Autodesk Inventor part; units mm, degrees
ref_plane "YZ Plane" through (0, 0, 0) normal (1, 0, 0) x (0, 1, 0)
ref_plane "XZ Plane" through (0, 0, 0) normal (0, 1, 0) x (-1, 0, 0)
ref_plane "XY Plane" through (0, 0, 0) normal (0, 0, 1) x (1, 0, 0)
sketch "Sketch1" plane through (0, 0, 0) normal (0, 0, 1) x (1, 0, 0)
  arc A0 (0, 12.7) -> (0, -12.7) centre (0, 0) ccw
  line L0 (0, 12.7) -> (17.145, 12.7)
  line L1 (17.145, 12.7) -> (17.145, -12.7)
  line L2 (17.145, -12.7) -> (0, -12.7)
  line L3 (0, -12.7) -> (0, 12.7)
  dimension "d0" = 25.4
  dimension "d7" = 17.145
extrude "Extrusion1" add sketch "Sketch1" along normal blind 4
sketch "Sketch2" plane through (0, 0, 4) normal (0, 0, 1) x (1, 0, 0)
  circle A0 centre (0, 0) radius 2.75
  dimension "d4" = 5.5
extrude "Extrusion2" cut sketch "Sketch2" against normal through all
sketch "Sketch3" plane through (17.145, -12.7, 0) normal (1, 0, 0) x (0, 0, -1)
  line L0 (-9.3431, 3.937) -> (-2.54, 3.937)
  line L1 (4.3638, 3.937) -> (4.3638, 21.463)
  line L2 (4.3638, 21.463) -> (0, 21.463)
  line L3 (-9.3431, 21.463) -> (-9.3431, 3.937)
  arc A0 (-2.54, 3.937) -> (0, 3.937) centre (-1.27, 3.937) ccw
  arc A1 (0, 21.463) -> (-2.54, 21.463) centre (-1.27, 21.463) ccw
  line L4 (0, 0) -> (0, 25.4)
  line L5 (-2.54, 3.937) -> (0, 3.937)
  line L6 (0, 3.937) -> (4.3638, 3.937)
  line L7 (0, 21.463) -> (-9.3431, 21.463)
  arc A2 (0, 3.937) -> (-2.54, 3.937) centre (-1.27, 3.937) ccw
  arc A3 (-2.54, 21.463) -> (0, 21.463) centre (-1.27, 21.463) ccw
  point P0 (0, 12.7)
  point P1 (4.3638, 12.7)
  point P2 (0, 12.7)
  dimension "d8" = 2.54
  dimension "d9" = 17.526
extrude "Extrusion3" cut sketch "Sketch3" against normal blind 8.89 contours L3 L7 A3 L4 A2 L0 | L4 L2 L1 L6
properties part number "fakebattergasket1"
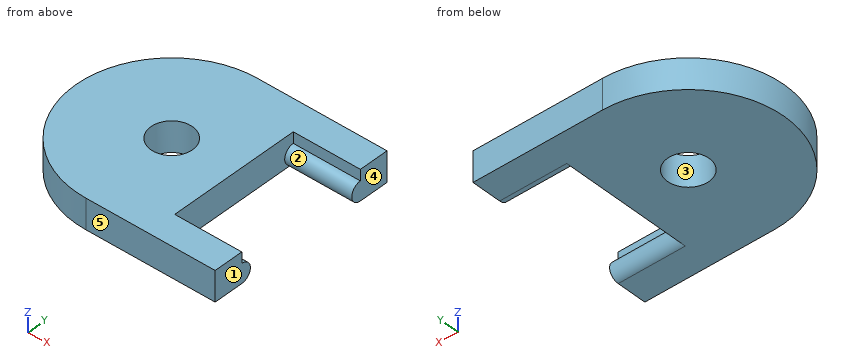
Model file for the job. Use its own axes, mm. Face numbers are marked on the shaded views. A direction names the side the tool comes from. Give positions to 0.01 mm unless a question says otherwise; leave off trailing zeros. Loops run counter-clockwise (first coordinate to the right, second up) from the corner with the lowest first, then second, coordinate; pieces in that order, holes last. Notation, with made-up numbers: (2.25, 22.25) -> (57.25, 22.25) arc R29 cw to (57.25, 53.25) -> close; hole circle Ø3 at (0.5, 27.25). An arc over 180 degrees is marked (long way). Use CSV: the item, a comma, the result in double quotes. Start each with the question number.
1) Slice it at C-C on z = 1.27. Give the cut face in (x, y) (3 decimals).
2) Mould opens along Y. For the marked faces 3, 4 and 5 say: released by +Y, released by -Y, zero draft, split by the parting line, or undercut.
3) Slice it at A-A on x = 13.25. Give the cut face in (y, z).
4) Flat gauge pin, fed straight in: pin 1 Ø2 at (y, z) = (2, 1.5) entering from +X (3 decimals). Where does the tip first touch, or does it go through?
5) Slice it at B-B on y = 0. Give the cut face in (x, z) (3 decimals), plus the area to 3 significant figures.
6) Wall check: line 1 (Y direction, x = 0, z = 1.55); line 2 (Y direction, x = 2, z = 3.4); line 3 (X direction, y = 2.25, z = 1.5) (3 decimals). Give the ranges that are in metal, low to high.
7) Slice it at D-D on y = -8. Give the cut face in (x, z) (3 decimals), plus the area to 3 significant figures.
8) Tool access for the marked faces 1 and 2: list every direction of +Z, -Z, +X, -X, +Y, -Y with a clear straight run to the whole face (end or side of a thin tool).
Computed values:
1,outline,"(0, -12.7) -> (17.145, -12.7) -> (17.145, -7.493) -> (8.255, -7.493) -> (8.255, 7.493) -> (17.145, 7.493) -> (17.145, 12.7) -> (0, 12.7) arc R12.7 ccw to start; hole circle Ø5.5 at (0, 0)"
2,face 3,"undercut"
2,face 4,"zero draft"
2,face 5,"released by -Y"
3,outline,"(-12.7, 0) -> (-8.76, 0) arc R1.27 ccw to (-8.76, 2.54) -> (-8.76, 4) -> (-12.7, 4) -> close; (8.76, 0) -> (12.7, 0) -> (12.7, 4) -> (8.76, 4) -> (8.76, 2.54) arc R1.27 ccw to start"
4,pin 1,"stops at x = 8.255"
5,outline,"(-12.7, 0) -> (-2.75, 0) -> (-2.75, 4) -> (-12.7, 4) -> close; (2.75, 0) -> (8.255, 0) -> (8.255, 4) -> (2.75, 4) -> close"
5,area,"61.8 mm^2"
6,line 1,"y = -12.7 to -2.75, 2.75 to 12.7"
6,line 2,"y = -12.7 to -1.89, 1.89 to 12.7"
6,line 3,"x = -12.499 to -1.581, 1.581 to 8.255"
7,outline,"(-9.864, 0) -> (8.255, 0) -> (8.255, 0.255) -> (17.145, 0.255) -> (17.145, 2.285) -> (8.255, 2.285) -> (8.255, 4) -> (-9.864, 4) -> close"
7,area,"90.5 mm^2"
8,face 1,"+Z, -Z, +X, +Y, -Y"
8,face 2,"+X"
